Autodesk Inventor part; units mm, degrees
ref_plane "YZ Plane" through (0, 0, 0) normal (1, 0, 0) x (0, 1, 0)
ref_plane "XZ Plane" through (0, 0, 0) normal (0, 1, 0) x (-1, 0, 0)
ref_plane "XY Plane" through (0, 0, 0) normal (0, 0, 1) x (1, 0, 0)
sketch "Sketch1" plane through (0, 0, 0) normal (0, 0, 1) x (1, 0, 0)
  line L0 (0, 0) -> (450, 0)
  line L1 (450, 0) -> (450, 100)
  line L2 (450, 100) -> (0, 100)
  line L3 (0, 100) -> (0, 0)
  line L4 (35, 40.5) -> (415, 40.5)
  line L5 (415, 40.5) -> (415, 55.5)
  line L6 (415, 55.5) -> (35, 55.5)
  line L7 (35, 55.5) -> (35, 40.5)
  circle A0 centre (35, 48) radius 7.5
  circle A1 centre (415, 48) radius 7.5
  point P0 (35, 40.5)
  point P1 (35, 55.5)
  dimension "d0" = 450
  dimension "d1" = 100
  dimension "d2" = 380
  dimension "d3" = 15
  dimension "d4" = 15
  dimension "d5" = 15
  dimension "d8" = 35
  dimension "d9" = 52
extrude "Extrusion1" add sketch "Sketch1" along normal blind 0.602
equation "\"BendRadius\" = Thickness"
equation "\"BendReliefWidth\" = Thickness"
equation "\"BendReliefDepth\" = 0.5 * Thickness"
equation "\"CornerReliefSize\" = 4 * Thickness"
equation "\"MinimumRemnant\" = 2 * Thickness"
equation "\"TransitionRadius\" = BendRadius"
equation "\"JacobiRadiusSize\" = BendRadius"
equation "\"GapSize\" = Thickness"
properties part number "project slit" material "Steel, Galvanized"
Geometry check sheet. Reference: the model listing, model coordinates, mm. A direction names the side the tool comes from. Give positions to 0.01 mm unless a question says otherwise; leave off trailing zeros. Loops run counter-clockwise (first coordinate to the right, second up) from the corner with the lowest first, then second, coordinate; pieces in that order, holes last. Notation, with made-up numbers: M 86,-21 L 120,-21 A25 ccw 120,10 Z; hole C 46.5,73.5 d2. An arc over 180 degrees is marked long. Write item = value, one per line.
(1) Sectioned sample at C-C, the plane z = 0.45. Record the cut outline in (x, y).
Answer below:
outline = M 0,0 L 450,0 L 450,100 L 0,100 Z; hole M 35,40.5 L 415,40.5 A7.5 ccw 415,55.5 L 35,55.5 A7.5 ccw Z
(2) Material ranges on line 1 (Y direction, x = 84, z = 0.3); line 2 (X direction, y = 50, z = 0.25), recorded low to high. Write a range as [from, to].
Answer below:
line_1 = [0, 40.5], [55.5, 100]
line_2 = [0, 27.77], [422.23, 450]
(3) Release check for a two-part mould opening along X. For faces 1 (the face through (222, 62, 0)), 2 (the face through (422.5, 48.16, 0.3)) record: released by +X, released by -X, zero draft, split by the parting line, or undercut.
Answer below:
face_1 = zero draft
face_2 = undercut
(4) Tool access check on faces 3 (the face through (27.5, 47.84, 0.3)), 4 (the face through (222, 62, 0.602)). Record the directions out of +Z, -Z, +X, -X, +Y, -Y that give a thin tool (end or side, any length) a straight path to the whole face; none if there is none.
Answer below:
face_3 = +Z, -Z
face_4 = +Z, +X, -X, +Y, -Y
(5) Sectioned sample at A-A, the plane x = 318. Record the cut outline in (y, z), plus the area to 3 significant figures.
Answer below:
outline = M 0,0 L 40.5,0 L 40.5,0.6 L 0,0.6 Z; M 55.5,0 L 100,0 L 100,0.6 L 55.5,0.6 Z
area = 51.2 mm2
(6) Sectioned sample at B-B, the plane y = 48. Record the cut outline in (x, z), plus the area to 3 significant figures.
Answer below:
outline = M 0,0 L 27.5,0 L 27.5,0.6 L 0,0.6 Z; M 422.5,0 L 450,0 L 450,0.6 L 422.5,0.6 Z
area = 33.1 mm2
